Input: part model. Units: mm. Frame: model coordinates. A direction names the side the tool comes from. Give positions to 0.01 mm unless a question says otherwise; leave off trailing zeros. Loops run counter-clockwise (first coordinate to the right, second up) from the corner with the lowest first, then second, coordinate; pieces in that order, holes last. Notation, with made-up numbers: M -19,9 L 28,9 A21 cw 28,36 Z; hole C 12.5,-33.5 d8. An arc over 180 degrees is marked long. Use CSV: the item, a comma, the result in double quotes. Start each with the question number.
from build123d import *

# Parameters (mm, degrees)
PAD_DEPTH      = 40
SKETCH001_R    = 1.65
HOLE_DEPTH     = 10
HOLE_TIPS_R    = 1.65
SKETCH002_R    = 1.65
HOLE001_DEPTH  = 12
HOLE001_TIPS_R = 1.65


with BuildPart() as part:
    # Sketch → Pad (new body)
    with BuildSketch(Plane.XY):
        Polygon((65, 0), (85, 0), (85, 4.4), (69.4, 20), (65, 20), align=None)
    extrude(amount=PAD_DEPTH)

    # Sketch001 (on Face1 of Pad) → Hole (cut)
    with BuildSketch(Plane.XZ):
        with Locations((75, 30)):
            Circle(SKETCH001_R)
        with Locations((75, 10)):
            Circle(SKETCH001_R)
    extrude(amount=-HOLE_DEPTH, mode=Mode.SUBTRACT)

    # Hole tips → Hole tip 1 section 0
    with BuildSketch(Plane.XZ.offset(-10), mode=Mode.PRIVATE) as hole_tip_1_s0:
        with Locations((75, 30)):
            Circle(HOLE_TIPS_R)
    loft([hole_tip_1_s0.sketch, Vertex(75, 10.99142, 30)], mode=Mode.SUBTRACT)

    # Hole tips → Hole tip 2 section 0
    with BuildSketch(Plane.XZ.offset(-10), mode=Mode.PRIVATE) as hole_tip_2_s0:
        with Locations((75, 10)):
            Circle(HOLE_TIPS_R)
    loft([hole_tip_2_s0.sketch, Vertex(75, 10.99142, 10)], mode=Mode.SUBTRACT)

    # Sketch002 (on Face4 of Hole) → Hole001 (cut)
    with BuildSketch(Plane.XY.offset(40)):
        with Locations((70, 10)):
            Circle(SKETCH002_R)
    extrude(amount=-HOLE001_DEPTH, mode=Mode.SUBTRACT)

    # Hole001 tips → Hole001 tip 1 section 0
    with BuildSketch(Plane.XY.offset(28), mode=Mode.PRIVATE) as hole001_tip_1_s0:
        with Locations((70, 10)):
            Circle(HOLE001_TIPS_R)
    loft([hole001_tip_1_s0.sketch, Vertex(70, 10, 27.00858)], mode=Mode.SUBTRACT)


solid = part.part
Item 1: Mould query, pull axis X, two halves, no side actions, for faces 4 (the flat face through (75, 0, 20)), 5 (the flat face through (85, 2, 20)), 6 (the conical face through (69.737, 10.012, 27.167)). Classes: +X half, -X half, draft (parallel to the pull), parting line (faces both ways), or undercut.
Item 2: Section A-A (z = 33). Output: boundary loops of the cut face in (x, y).
Item 3: Section B-B (y = 5). Output: boundary loops of the cut face in (x, z), then the cut area to 3 significant figures.
Item 4: Section D-D (x = 77.75). Output: boundary loops of the cut face in (y, z), then the cut area to 3 significant figures.
Item 5: Material intervals for line 1 (Z direction, x = 75, y = 6.5); line 2 (Z direction, x = 75.75, y = 9.25); line 3 (Y direction, x = 70, z = 35.5), sorted ascending.
Item 6: Set-up query: faces 1 (the cylindrical face through (68.35, 10.07, 34.08)), 2 (the flat face through (77.3, 12.1, 19.7)), 3 (the cylindrical face through (73.784, 4.93, 31.115)). Return all of +Z, -Z, +X, -X, +Y, -Y with unobstructed straight access to the full face (end or side cutting, diameter ignored); none if empty.
Item 7: Section C-C (z = 4.5). Output: boundary loops of the cut face in (x, y), then the cut area to 3 significant figures.
Item 8: First-contact query: pin 1 Ø2 at (y, z) = (9, 6.5) entering from +X; pin 2 Ø2 at (x, z) = (75, 30) entering from +Y; pin 3 Ø2 at (x, z) = (75, 10) entering from -Y. Flat tips, straight axial feed; report the tip coordinate or a pass-through.
Recorded:
1,face 4,"draft"
1,face 5,"+X half"
1,face 6,"undercut"
2,outline,"M 65,0 L 85,0 L 85,4.4 L 69.4,20 L 65,20 Z; hole C 70,10 d3.3"
3,outline,"M 65,0 L 84.4,0 L 84.4,40 L 65,40 Z; hole C 75,10 d3.3; hole C 75,30 d3.3"
3,area,"759 mm²"
4,outline,"M 0,0 L 11.65,0 L 11.65,40 L 0,40 Z"
4,area,"466 mm²"
5,line 1,"0 to 8.35, 11.65 to 28.35, 31.65 to 40"
5,line 2,"0 to 8.53, 11.47 to 28.53, 31.47 to 40"
5,line 3,"0 to 8.35, 11.65 to 19.4"
6,face 1,"+Z"
6,face 2,"+Z, -Z, +X, +Y"
6,face 3,"-Y"
7,outline,"M 65,0 L 85,0 L 85,4.4 L 69.4,20 L 65,20 Z"
7,area,"278 mm²"
8,pin 1,"x = 81.4"
8,pin 2,"y = 15.4"
8,pin 3,"y = 10.39"
